Job drawing, mm, ordinate dimensions from the low corner. One solid piece. Give positions to 0.01 mm unless a question says otherwise; leave off trailing zeros. Order: outer loops, then holes, each group sorted by start corner. A loop starts at its lowest first (then second) coordinate and runs counter-clockwise, first axis right, second up. Notation, with made-up numbers: (-2.75, 22) -> (13.25, 22) arc R23 ccw to (13.25, 56) -> close; hole circle Ø3 at (44, 50.25). An arc over 180 degrees is marked (long way). Write item = value, one per line. Start each with the question number.
(1) Probe line 1 along Z through (x, y) = (28.5, 8) (1 decimal); line 2 along Z through (x, y) = (25, 2); line 3 along X through (y, z) = (19.5, 30.5) (1 decimal). List the from-to ranges inside material, lowest first. Write a range as from..to.
(2) Two-plate mould, pull along Z, no slides. Class the marked faces 1, 2, 3 and 4: pulls with the +Z half, pulls with the -Z half, needs draft (parallel to the pull), parting line crosses it, or undercut.
(3) Saw through at B-B, the plane y = 6.5. List the corners of the cut face in (x, z), then the cut area to 3 significant figures.
(4) Flat gauge pin, fed straight in: pin 1 (6 mm diameter, centred on x = 27.11, z = 27.41, fed in from +Y). Where does the tip first touch, or does it go through?
(5) Saw through at A-A, the plane x = 28.5. List the corners of the cut face in (y, z) (1 decimal), then the cut area to 3 significant figures.
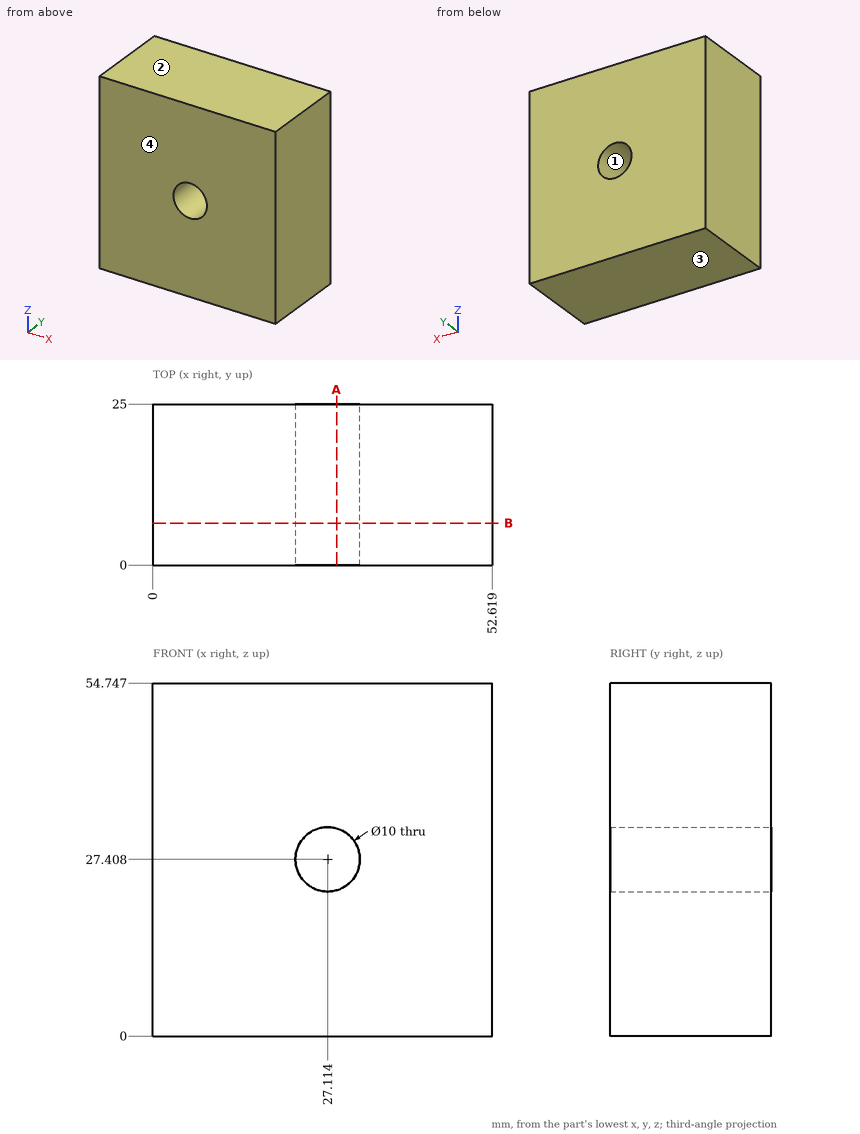
Results list:
q1.line_1 = 0..22.6, 32.2..54.7
q1.line_2 = 0..22.88, 31.94..54.75
q1.line_3 = 0..23.2, 31..52.6
q2.face_1 = undercut
q2.face_2 = pulls with the +Z half
q2.face_3 = pulls with the -Z half
q2.face_4 = needs draft
q3.outline = (0, 0) -> (52.62, 0) -> (52.62, 54.75) -> (0, 54.75) -> close; hole circle Ø10 at (27.11, 27.41)
q3.area = 2,800 mm^2
q4.pin_1 = through
q5.outline = (0, 0) -> (25, 0) -> (25, 22.6) -> (0, 22.6) -> close; (0, 32.2) -> (25, 32.2) -> (25, 54.7) -> (0, 54.7) -> close
q5.area = 1,130 mm^2
